Geometry check sheet. Reference: drawing and pictorial views, mm from the part's lowest x, y, z. A direction names the side the tool comes from. Give positions to 0.01 mm unless a question says otherwise; leave off trailing zeros. Write each loop counter-clockwise with the first axis right and the second up, starting at its lowest first coordinate (ties: lowest second). Pieces come first, ordered by that corner, then holes. Notation, with made-up numbers: (-9.5, -9.75) -> (48.5, -9.75) arc R23 cw to (48.5, 20.25) -> close; hole circle Ø3 at (8, 25.25). An arc over 180 degrees is marked (long way). Use a Markdown table: item, result. Add a question column.
1. Cross-section at A-A (x = 2). Enter the section's corners in (y, z), then the cut area to 3 significant figures.
2. Cross-section at B-B (y = 7). Enter the section's corners in (x, z), then the cut area to 3 significant figures.
3. Gauge pin test, flat ends, axial feed: P1, Ø1.5, axis at y = 5, z = 2, coming from the +X side; P2, Ø1.5, axis at x = 9.5, z = 3, coming from the -Y side. Record the tip position at first contact, or that the pin passes through.
4. Set-up check for the marked faces 1 and 2: record each of +Z, -Z, +X, -X, +Y, -Y from which the full face is reachable in a straight line by a thin tool's end or side.
5. Cross-section at C-C (z = 0.45). Enter the section's corners in (x, y) (3 decimals), then the cut area to 3 significant figures.
6. Scan lines: probe 1 along Y at (x, z) = (9, 3.75); probe 2 along X at (y, z) = (8, 4); probe 3 along Y at (x, z) = (4, 2.6). Record each from-to range of solid material in increasing order. Write a range as [from, to].
7. Cross-section at D-D (x = 6). Enter the section's corners in (y, z).
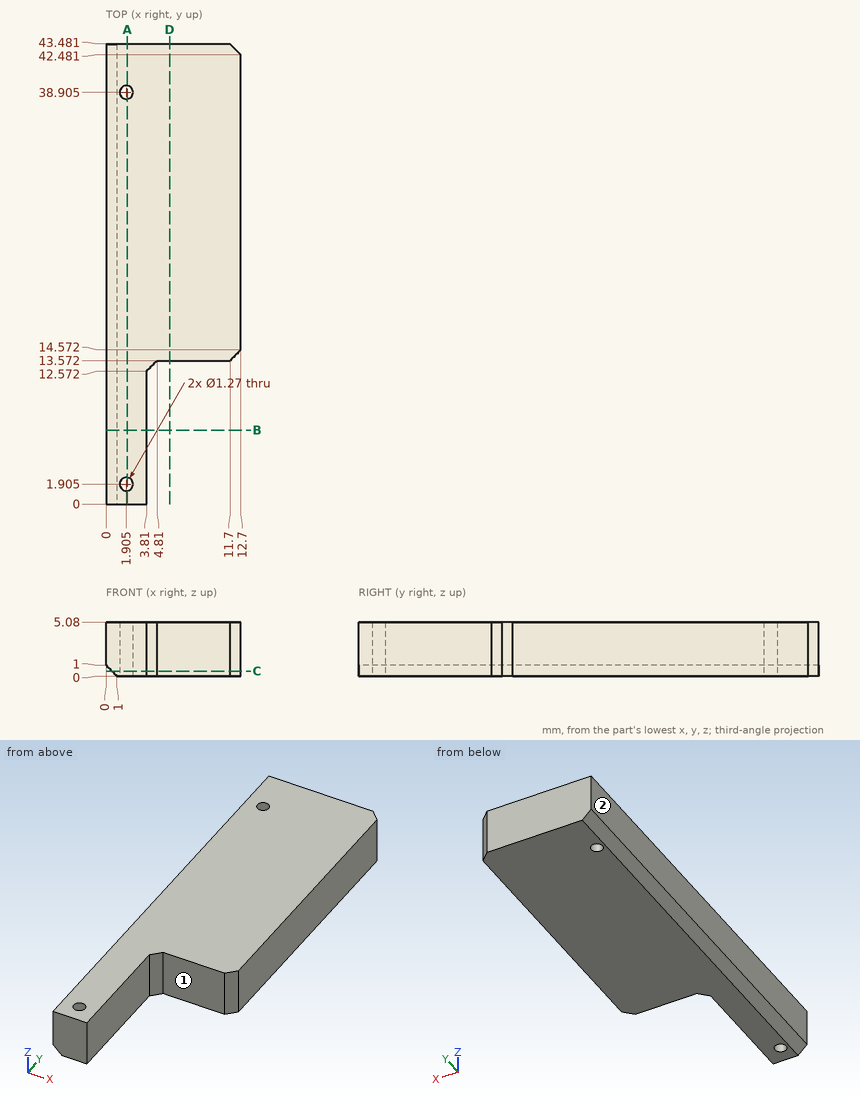
Worked answers:
| question | item | result |
|---|---|---|
| 1 | outline | (0, 0) -> (1.28, 0) -> (1.28, 5.08) -> (0, 5.08) -> close; (2.53, 0) -> (38.28, 0) -> (38.28, 5.08) -> (2.53, 5.08) -> close; (39.53, 0) -> (43.48, 0) -> (43.48, 5.08) -> (39.53, 5.08) -> close |
| 1 | area | 208 mm² |
| 2 | outline | (0, 1) -> (1, 0) -> (3.81, 0) -> (3.81, 5.08) -> (0, 5.08) -> close |
| 2 | area | 18.9 mm² |
| 3 | P1 | stops at x = 3.81 |
| 3 | P2 | stops at y = 13.57 |
| 4 | face 1 | +Z, -Z, +X, -Y |
| 4 | face 2 | +Z, -Z, -X, +Y, -Y |
| 5 | outline | (0.55, 0) -> (3.81, 0) -> (3.81, 12.572) -> (4.81, 13.572) -> (11.7, 13.572) -> (12.7, 14.572) -> (12.7, 42.481) -> (11.7, 43.481) -> (0.55, 43.481) -> close; hole circle Ø1.27 at (1.905, 1.905); hole circle Ø1.27 at (1.905, 38.905) |
| 5 | area | 405 mm² |
| 6 | probe 1 | y = [13.57, 43.48] |
| 6 | probe 2 | x = [0, 3.81] |
| 6 | probe 3 | y = [12.76, 43.48] |
| 7 | outline | (13.57, 0) -> (43.48, 0) -> (43.48, 5.08) -> (13.57, 5.08) -> close |
